Geometry: final body of the model. Coordinates: model frame, mm. A direction names the side the tool comes from. Give positions to 0.01 mm unless a question says otherwise; leave off trailing zeros. Order: outer loops, then holes, each group sorted by start corner. A loop starts at its lowest first (then second) coordinate and runs counter-clockwise, first axis right, second up. Notation, with made-up numbers: (-6.75, 57.25) -> (9.25, 57.25) arc R18 cw to (9.25, 69.25) -> close; hole circle Ø9 at (-20.75, 76). An arc over 180 degrees is marked (long way). Write item = value, one per line.
```python
from build123d import *

# Parameters (mm, degrees)
BOSS_EXTRUDE1_DEPTH     = 100
CUT_EXTRUDE3_DEPTH      = 150
CUT_EXTRUDE3_DEPTH_BACK = 150
CUT_EXTRUDE6_DEPTH      = 150
CUT_EXTRUDE6_DEPTH_BACK = 150
FILLET7_R               = 8
SKETCH5_R               = 2.3
CUT_EXTRUDE7_DEPTH      = 5
SKETCH6_R               = 4.5
CUT_EXTRUDE8_DEPTH      = 150


with BuildPart() as part:
    # Sketch1 → Boss-Extrude1 (new body)
    with BuildSketch(Plane(origin=(0, 0, 0), x_dir=(0, 0, -1), z_dir=(1, 0, 0))):
        Polygon((-30, 27.8), (30, 27.8), (30, -27.8), (30, -57.8), (-62, -57.8), (-62, -27.8), (-62, 27.8), align=None)
    extrude(amount=BOSS_EXTRUDE1_DEPTH)

    # Sketch3 → Cut-Extrude3 (cut, two sides: drawn at the far end of the back side and taken through both)
    with BuildSketch(Plane(origin=(0, 0, 0), x_dir=(1, 0, 0), z_dir=(0, 1, 0)).offset(-CUT_EXTRUDE3_DEPTH_BACK)):
        Polygon((0, 30), (100, -16), (100, 30), align=None)
        Polygon((100, -62), (0, -62), (0, -30), align=None)
    extrude(amount=CUT_EXTRUDE3_DEPTH + CUT_EXTRUDE3_DEPTH_BACK, mode=Mode.SUBTRACT)

    # Sketch4 → Cut-Extrude6 (cut, two sides: drawn at the far end of the back side and taken through both)
    with BuildSketch(Plane.XY.offset(-CUT_EXTRUDE6_DEPTH_BACK)):
        with BuildLine():
            Line((100, 27.8), (0, 27.8))
            add(Edge.make_bspline(
                [(0, 27.8), (55.001263305, 9.951718706), (100, -22.2)],
                knots=[0, 0, 0, 0.534302679, 0.534302679, 0.534302679], degree=2))
            Line((100, -22.2), (100, 27.8))
        make_face()
        with BuildLine():
            Line((0, -27.8), (0, -57.8))
            Line((0, -57.8), (100, -57.8))
            add(Edge.make_bspline(
                [(0, -27.8), (59.172869478, -28.215423473), (100, -57.8)],
                knots=[0, 0, 0, 0.618763152, 0.618763152, 0.618763152], degree=2))
        make_face()
    extrude(amount=CUT_EXTRUDE6_DEPTH + CUT_EXTRUDE6_DEPTH_BACK, mode=Mode.SUBTRACT)

    # Fillet7
    fillet7_edges = [part.edges().sort_by_distance(p)[0] for p in [
        (100, -40, 62),
        (100, -40, 16),
    ]]
    fillet(fillet7_edges, radius=FILLET7_R)

    # Sketch5 → Cut-Extrude7 (cut)
    with BuildSketch(Plane.ZY):
        with Locations((0, -5)):
            Circle(SKETCH5_R)
        with Locations((0, -25)):
            Circle(SKETCH5_R)
    extrude(amount=-CUT_EXTRUDE7_DEPTH, mode=Mode.SUBTRACT)

    # Sketch6 → Cut-Extrude8 (cut)
    with BuildSketch(Plane.ZY.offset(-5)):
        with Locations((0, -5)):
            Circle(SKETCH6_R)
        with Locations(Location((0, -25, 0), (0, 0, 320.073904161))):
            Circle(SKETCH6_R)
    extrude(amount=-CUT_EXTRUDE8_DEPTH, mode=Mode.SUBTRACT)


solid = part.part
```
1) First-contact query: P1, Ø12, axis at x = 49, y = -39, coming from the -Z side; P2, Ø10.5, axis at y = -25, z = 0, coming from the +X side; P3, Ø10, axis at x = 33, z = 17, coming from the -Y side; P4, Ø7, axis at y = -5, z = 0, coming from the -X side. Flat tips, straight axial feed; report the tip coordinate or a pass-through.
Check sheet entries:
P1 = -8.44
P2 = 76.63
P3 = -31.43
P4 = 0
2) Section query A-A (y = -25). Output: boundary loops of the cut face in (x, z), plus the area to 3 significant figures.
Check sheet entries:
outline = (0, -30) -> (55.43, -4.5) -> (5, -4.5) -> (5, -2.3) -> (0, -2.3) -> close; (0, 2.3) -> (5, 2.3) -> (5, 4.5) -> (75, 4.5) -> (95.34, 13.86) arc R8 ccw to (100, 21.13) -> (100, 51.04) arc R8 ccw to (89.56, 58.66) -> (0, 30) -> close
area = 4,700 mm²
3) Line query: line 1 (Y direction, x = 3.7, z = 0); line 2 (Z direction, x = 26, y = -25); line 3 (Z direction, x = 41, y = -6). Output: solid intervals per line, ascending. Write a range as from..to.
Check sheet entries:
line_1 = -27.85..-27.3, -22.7..-7.3, -2.7..26.58
line_2 = -18.04..-4.5, 4.5..38.32
line_3 = -11.14..-4.39, 4.39..43.12
4) Reachability of faces 1 (the face through (44.15, -12.1, 44.13)), 2 (the face through (5, -7, 2)) from +Z, -Z, +X, -X, +Y, -Y: full face, straight path, thin tool, end or side. Return the list, or none.
Check sheet entries:
face_1 = +Z, -X, +Y, -Y
face_2 = +X
5) Mould query, pull axis Y, two halves, no side actions, for faces 3 (the face through (98.701, -38.093, 16.756)), 4 (the face through (5, -22, 0)). Classes: +Y half, -Y half, draft (parallel to the pull), parting line (faces both ways), or undercut.
Check sheet entries:
face_3 = draft
face_4 = undercut
6) Section query B-B (x = 40). Count the separate pieces of the cut face and the enclosed holes in it, plus the area to 3 significant figures.
Check sheet entries:
separate_pieces = 1
enclosed_holes = 2
area = 2,280 mm²
